```python
from build123d import *

# Parameters (mm, degrees)
ESQUISSE1_R             = 7
BOSS_EXTRU_1_DEPTH      = 3
ESQUISSE2_R             = 5
BOSS_EXTRU_2_DEPTH      = 5
ESQUISSE3_R             = 2
ENL_V_MAT_EXTRU_1_DEPTH = 9
CONG_1_R                = 1
CHANFREIN1_SIZE         = 1
CHANFREIN1_SIZE2        = 0.176326981


with BuildPart() as part:
    # Esquisse1 → Boss.-Extru.1 (new body)
    with BuildSketch(Plane.XY):
        Circle(ESQUISSE1_R)
    extrude(amount=BOSS_EXTRU_1_DEPTH)

    # Esquisse2 → Boss.-Extru.2 (add)
    with BuildSketch(Plane.XY.offset(3)):
        Circle(ESQUISSE2_R)
    extrude(amount=BOSS_EXTRU_2_DEPTH)

    # Esquisse3 → Enlèv. mat.-Extru.1 (cut, through all)
    with BuildSketch(Plane.XY.offset(8)):
        Circle(ESQUISSE3_R)
    extrude(amount=-ENL_V_MAT_EXTRU_1_DEPTH, mode=Mode.SUBTRACT)

    # Congé1
    cong_1_edges = [part.edges().sort_by_distance(p)[0] for p in [
        (-5, 0, 3),
    ]]
    fillet(cong_1_edges, radius=CONG_1_R)

    # Chanfrein1
    chanfrein1_edges = [part.edges().sort_by_distance(p)[0] for p in [
        (-5, 0, 8),
    ]]
    chanfrein1_side = [part.faces().sort_by_distance(p)[0] for p in [
        (-4.858578644, 0, 8),
    ]]
    chamfer(chanfrein1_edges, length=CHANFREIN1_SIZE, length2=CHANFREIN1_SIZE2, reference=chanfrein1_side[0])


solid = part.part
```
The model under review builds one solid part; all positions refer to its coordinate system, in mm. Round coordinates to 2 decimals unless told otherwise and drop trailing zeros. Loops run counter-clockwise (first coordinate to the right, second up) from the corner with the lowest first, then second, coordinate; pieces in that order, holes last.
Item 1: Take a section at D-D (z = 5). Write out the cut boundary in (x, y).
Determined:
outline: circle Ø10 at (0, 0); hole circle Ø4 at (0, 0)
Item 2: Take a section at C-C (z = 0.5). Write out the cut boundary in (x, y).
Determined:
outline: circle Ø14 at (0, 0); hole circle Ø4 at (0, 0)
Item 3: For line 1 (Y direction, x = 0, z = 6); line 2 (Y direction, x = 0, z = 1.5); line 3 (Z direction, x = -1, y = -6.5), list the stretches that pass through material, from the lowest coordinate up.
Determined:
line 1: y = -5 to -2, 2 to 5
line 2: y = -7 to -2, 2 to 7
line 3: z = 0 to 3
Item 4: Mouldability with a two-part tool opening along Y and no side actions: class faces 1 (the face through (-1.08, -4.88, 5.89)), 2 (the face through (6, 2, 3)), 3 (the face through (0, -2, 4)) as released by +Y, released by -Y, zero draft, split by the parting line, or undercut.
Determined:
face 1: split by the parting line
face 2: zero draft
face 3: undercut
Item 5: Clearance check with flat-ended pins moving along their axes: pin 1 Ø4 at (y, z) = (3, 1) entering from -X; pin 2 Ø3 at (x, y) = (3, 3.5) entering from -Z; pin 3 Ø2 at (y, z) = (2.5, 5) entering from -X; pin 4 Ø1.5 at (y, z) = (5, 4.5) entering from -X. State where each tip first meets the part, or that it passes through.
Determined:
pin 1: stops at x = -6.93
pin 2: stops at z = 0
pin 3: stops at x = -4.77
pin 4: stops at x = -2.63
Item 6: Take a section at A-A (y = 0). Write out the cut boundary in (x, z).
Determined:
outline: (-7, 0) - (-2, 0) - (-2, 8) - (-4, 8) - (-5, 7.82) - (-5, 4) arc R1 cw to (-6, 3) - (-7, 3) - close; (2, 0) - (7, 0) - (7, 3) - (6, 3) arc R1 cw to (5, 4) - (5, 7.82) - (4, 8) - (2, 8) - close
